CAD build for the part. Positions are in the model's coordinates, mm. Give positions to 0.01 mm unless a question says otherwise; leave off trailing zeros. Loops run counter-clockwise (first coordinate to the right, second up) from the corner with the lowest first, then second, coordinate; pieces in that order, holes last.
Item 1: Probe probe 1 along Y at (x, z) = (1135.75, 195) (3 decimals); probe 2 along X at (y, z) = (4.5, -320.5); probe 3 along Y at (x, z) = (1124.75, -461). List the from-to ranges inside material, lowest first.
Item 2: Drop flat-ended pins along their axis: P1, Ø4, axis at x = 1133.5, y = 32, coming from the -Z side; P2, Ø8, axis at x = 1125, y = 30.5, coming from the +Z side; P3, Ø1.5, axis at y = 22.5, z = 381.5, coming from the -X side; P4, Ø5, axis at x = 1136.5, z = 291, coming from the -Y side. Give the stop position or say it passes through.
Item 3: Saw through at B-B on x = 1133.25. Give the cut face in (y, z) (3 decimals), plus the area to 3 significant figures.
from build123d import *

# Parameters (mm, degrees)
EXTRUDE1_DEPTH     = 542.13125
CUT_EXTRUDE1_DEPTH = 25.4
CUT_EXTRUDE2_DEPTH = 25.4


with BuildPart() as part:
    # Sketch1 → Extrude1 (new body, symmetric)
    with BuildSketch(Plane.XY):
        with BuildLine():
            Line((1143, 0), (1142.20625, 0))
            Line((1142.20625, 0), (1142.20625, 32.54375))
            ThreePointArc((1142.20625, 32.54375), (1141.741282015, 33.666282015), (1140.61875, 34.13125))
            Line((1140.61875, 34.13125), (1128.140506397, 34.13125))
            Line((1128.140506397, 34.13125), (1123.091401986, 31.071186722))
            Line((1123.091401986, 31.071186722), (1122.68, 31.75))
            Line((1122.68, 31.75), (1127.91875, 34.925))
            Line((1127.91875, 34.925), (1140.61875, 34.925))
            ThreePointArc((1140.61875, 34.925), (1142.302548023, 34.227548023), (1143, 32.54375))
            Line((1143, 32.54375), (1143, 0))
        make_face()
    extrude(amount=EXTRUDE1_DEPTH, both=True)

    # Sketch2 → Cut-Extrude1 (cut)
    with BuildSketch(Plane(origin=(1143, 0, 0), x_dir=(0, 0, -1), z_dir=(1, 0, 0))):
        Polygon((542.13125, 34.925), (484.98125, 34.925), (484.98125, 31.75), (542.13125, 20.6502), align=None)
    extrude(amount=-CUT_EXTRUDE1_DEPTH, mode=Mode.SUBTRACT)

    # Sketch3 → Cut-Extrude2 (cut)
    with BuildSketch(Plane(origin=(0, 0, -484.98125), x_dir=(-1, 0, 0), z_dir=(0, 0, -1))):
        Polygon((-1127.91875, 34.925), (-1122.68, 31.75), (-1123.420434334, 30.528283348), (-1128.140506397, 34.13125), align=None)
    extrude(amount=CUT_EXTRUDE2_DEPTH, mode=Mode.SUBTRACT)


solid = part.part
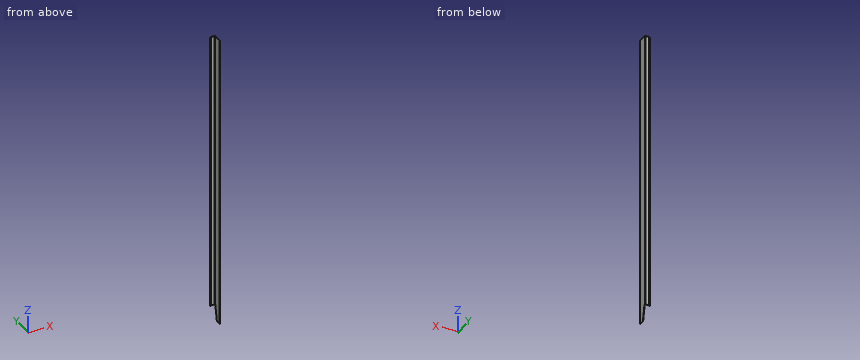
Results below:
1. probe 1: y = 34.131 to 34.925
1. probe 2: x = 1142.21 to 1143
1. probe 3: y = 32.08 to 33
2. P1: passes through
2. P2: stops at z = 542.13
2. P3: stops at x = 1142.21
2. P4: stops at y = 34.13
3. outline: (34.131, -484.981) - (34.925, -484.981) - (34.925, 542.131) - (34.131, 542.131) - close
3. area: 815 mm2
